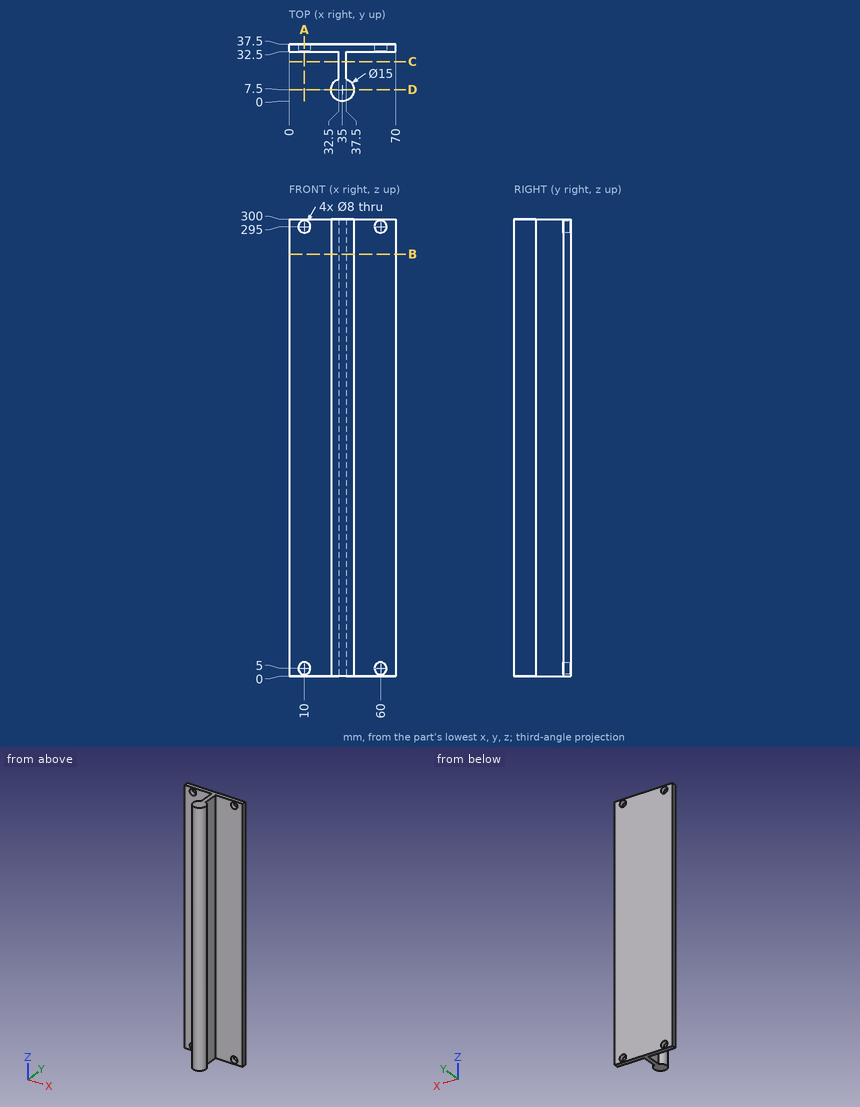
Source: three-view drawing plus pictorial views. Frame: mm from the lowest corner of the part. Give positions to 0.01 mm unless a question says otherwise; leave off trailing zeros. Loops run counter-clockwise (first coordinate to the right, second up) from the corner with the lowest first, then second, coordinate; pieces in that order, holes last. Notation, with made-up numbers: M 49.25,19 L 64.25,19 A21 cw 64.25,39 Z; hole C -5,28.5 d8. An arc over 180 degrees is marked long. Use CSV: the item, a comma, the result in double quotes.
(1) Pin query (flat end, axial travel): P1, Ø5, axis at y = 16.5, z = 260.5, coming from the -X side; P2, Ø1.5, axis at y = 21.5, z = 235, coming from the -X side; P3, Ø10, axis at y = 10.5, z = 255.5, coming from the -X side; P4, Ø12, axis at y = 27, z = 73.5, coming from the -X side. Return the tip coordinate at first contact, or that it passes through.
Outcome:
P1,"stops at x = 31.26"
P2,"stops at x = 32.5"
P3,"stops at x = 27.5"
P4,"stops at x = 0"
(2) Section A-A, the plane x = 10. Return loops of the section in (y, z), plus the area to 3 significant figures.
Outcome:
outline,"M 32.5,0 L 37.5,0 L 37.5,1 L 32.5,1 Z; M 32.5,9 L 37.5,9 L 37.5,291 L 32.5,291 Z; M 32.5,299 L 37.5,299 L 37.5,300 L 32.5,300 Z"
area,"1,420 mm²"
(3) Material intervals for L1, parallel to X at y = 33, z = 295; L2, parallel to Z at x = 10, y = 36; L3, parallel to X at y = 15.5, z = 104, sorted ascending. Write a range as [from, to].
Outcome:
L1,"x = [0, 6], [14, 56], [64, 70]"
L2,"z = [0, 1], [9, 291], [299, 300]"
L3,"x = [32.5, 37.5]"
(4) Section C-C, the plane y = 26. Return loops of the section in (x, z).
Outcome:
outline,"M 32.5,0 L 37.5,0 L 37.5,300 L 32.5,300 Z"
(5) Section D-D, the plane y = 7.5. Return loops of the section in (x, z).
Outcome:
outline,"M 27.5,0 L 42.5,0 L 42.5,300 L 27.5,300 Z"
(6) Section B-B, the plane z = 277. Return loops of the section in (x, y), plus the area to 3 significant figures.
Outcome:
outline,"M 0,32.5 L 32.5,32.5 L 32.5,14.57 A7.5 ccw long 37.5,14.57 L 37.5,32.5 L 70,32.5 L 70,37.5 L 0,37.5 Z"
area,"615 mm²"
